Geometry: final body of the model. Coordinates: model frame, mm. Give positions to 0.01 mm unless a question says otherwise; leave off trailing zeros. Order: outer loops, then holes, each group sorted by start corner. A loop starts at its lowest first (then second) coordinate and runs counter-clockwise, first axis right, second up. Notation, with made-up numbers: (-36.5, 46.5) - (-21.5, 46.5) arc R30 cw to (-21.5, 73.5) - close; hole circle Ø11 at (27.25, 18). An arc over 180 degrees is marked (long way). Put each result on its own line as item: value. Start each with the question number.
1. First-contact query: P1, Ø1.5, axis at x = 20, y = 1, coming from the -Z side. Flat tip, straight axial feed; report the tip coordinate or a pass-through.
2. Section A-A on x = 20. Return the cut outline in (y, z) (3 decimals), plus the area to 3 significant figures.
3. Section B-B on z = -6. Return the cut outline in (x, y) (3 decimals).
4. Ray query, line 1 along Z through (x, y) = (-13, 1.5); line 2 along X through (y, z) = (1.45, 5.5); line 3 along Z through (x, y) = (55.5, 2.75). Return the intervals inside material, ascending. Write a range as from..to.
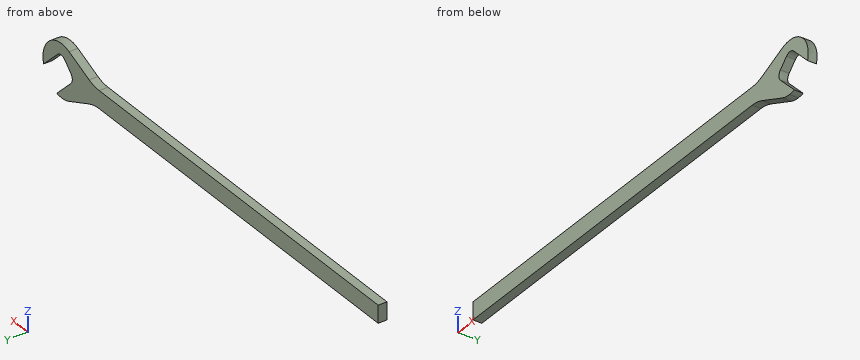
from build123d import *

# Parameters (mm, degrees)
BOSS_EXTRUDE1_DEPTH = 3.175


with BuildPart() as part:
    # Sketch1 → Boss-Extrude1 (new body)
    with BuildSketch(Plane(origin=(0, 0, 0), x_dir=(1, 0, 0), z_dir=(0, 1, 0))):
        with BuildLine():
            Line((1.259536023, 2.586263405), (-100.340463977, 2.586263405))
            Line((-100.340463977, 2.586263405), (-103.395029965, 2.586263405))
            Line((-103.395029965, 2.586263405), (-103.395029965, -3.763736604))
            Line((-103.395029965, -3.763736604), (39.35953602, -3.763736604))
            add(Edge.make_bspline(
                [(39.35953602, -3.763736604), (40.672498996, -3.763736604), (41.958231282, -4.032454171), (43.243430957, -4.301060422), (44.446955668, -4.827235355)],
                knots=[0, 0, 0, 0.5, 0.5, 1, 1, 1], degree=2))
            Line((44.446955668, -4.827235355), (54.714405304, -9.316112529))
            add(Edge.make_bspline(
                [(54.714405304, -9.316112529), (55.946669165, -9.854852073), (57.28046692, -10.031425137), (58.61345219, -10.207890641), (59.944261722, -10.008152925), (61.273983438, -9.808578475), (62.497433966, -9.248116189), (63.719884433, -8.68811203), (64.740280541, -7.810763211), (65.759842568, -6.934131546), (66.497371281, -5.80852035), (67.234297131, -4.683829239), (67.631270692, -3.397998317), (68.027919764, -2.113218446), (68.053287839, -0.767742461), (68.078640466, 0.576914214), (67.730413535, 1.876514813)],
                knots=[0, 0, 0, 0.125, 0.125, 0.25, 0.25, 0.375, 0.375, 0.5, 0.5, 0.625, 0.625, 0.75, 0.75, 0.875, 0.875, 1, 1, 1], degree=2))
            Line((67.730413535, 1.876514813), (60.546208639, -5.307690084))
            add(Edge.make_bspline(
                [(60.546208639, -5.307690084), (60.189154092, -5.664744631), (59.722173333, -5.858292872), (59.255944804, -6.051529339), (58.750157415, -6.05163886), (58.245470025, -6.051748143), (57.778141496, -5.858292872), (57.311565034, -5.665148928), (56.954106191, -5.307690084)],
                knots=[0, 0, 0, 0.25, 0.25, 0.5, 0.5, 0.75, 0.75, 1, 1, 1], degree=2))
            Line((56.954106191, -5.307690084), (53.811016549, -2.164600442))
            add(Edge.make_bspline(
                [(53.811016549, -2.164600442), (53.453962002, -1.807545895), (53.26041376, -1.340565136), (53.067177294, -0.874336608), (53.067067773, -0.368549218), (53.06695849, 0.136138171), (53.26041376, 0.6034667), (53.453557705, 1.070043162), (53.811016549, 1.427502006)],
                knots=[0, 0, 0, 0.25, 0.25, 0.5, 0.5, 0.75, 0.75, 1, 1, 1], degree=2))
            Line((53.811016549, 1.427502006), (60.995221446, 8.611706903))
            ThreePointArc((60.995221446, 8.611706903), (59.773232018, 8.854775714), (58.529970033, 8.93626341))
            ThreePointArc((58.529970033, 8.93626341), (56.580948585, 8.734725234), (54.714405295, 8.138639345))
            Line((54.714405295, 8.138639345), (44.446955671, 3.649762156))
            add(Edge.make_bspline(
                [(44.446955671, 3.649762156), (43.243940291, 3.1238099), (41.958231285, 2.854980972), (40.67305488, 2.586263405), (39.359536023, 2.586263405)],
                knots=[0, 0, 0, 0.5, 0.5, 1, 1, 1], degree=2))
            Line((39.359536023, 2.586263405), (1.259536023, 2.586263405))
        make_face()
    extrude(amount=BOSS_EXTRUDE1_DEPTH)


solid = part.part
Resolved:
1. P1: z = -2.59
2. outline: (0, -2.586) - (3.175, -2.586) - (3.175, 3.764) - (0, 3.764) - close
2. area: 20.2 mm^2
3. outline: (49.823, 0) - (58.384, 0) - (58.384, 3.175) - (49.823, 3.175) - close
4. line 1: -2.59..3.76
4. line 2: 45.99..57.17, 60.33..66.69
4. line 3: -8.44..-3.12, 3.85..9.62
